The listing builds one solid part. Answer for the finished solid, in the listing's coordinates (mm). A direction names the side the tool comes from. Coordinates: 2 decimals unless noted, no trailing zeros. Write each loop counter-clockwise with the first axis right and the second up, starting at its lowest first coordinate (ties: lowest second). Pieces come first, ordered by that corner, then holes.
from build123d import *

# Parameters (mm, degrees)
SKETCH1_W             = 32
SKETCH1_H             = 32
BOSS_EXTRUDE1_DEPTH   = 4
SKETCH2_R             = 2
CUT_EXTRUDE1_DEPTH    = 3
CHAMFER1_SIZE         = 2
CHAMFER1_SIZE2        = 1.154700538
CHAMFER1_PART_2_SIZE  = 2
CHAMFER1_PART_2_SIZE2 = 1.154700538
CHAMFER1_PART_3_SIZE  = 2
CHAMFER1_PART_3_SIZE2 = 1.154700538
CHAMFER1_PART_4_SIZE  = 2
CHAMFER1_PART_4_SIZE2 = 1.154700538


with BuildPart() as part:
    # Sketch1 → Boss-Extrude1 (new body)
    with BuildSketch(Plane(origin=(0, 0, 0), x_dir=(1, 0, 0), z_dir=(0, 1, 0))):
        Rectangle(SKETCH1_W, SKETCH1_H)
    extrude(amount=BOSS_EXTRUDE1_DEPTH)

    # Sketch2 → Cut-Extrude1 (cut)
    with BuildSketch(Plane(origin=(0, 4, 0), x_dir=(1, 0, 0), z_dir=(0, 1, 0))):
        with Locations((-11.75, 11.75)):
            Circle(SKETCH2_R)
        with Locations((11.75, 11.75)):
            Circle(SKETCH2_R)
        with Locations((11.75, -11.75)):
            Circle(SKETCH2_R)
        with Locations((-11.75, -11.75)):
            Circle(SKETCH2_R)
    extrude(amount=-CUT_EXTRUDE1_DEPTH, mode=Mode.SUBTRACT)

    # Chamfer1
    chamfer1_edges = [part.edges().sort_by_distance(p)[0] for p in [
        (-16, 4, 0),
    ]]
    chamfer1_side = [part.faces().sort_by_distance(p)[0] for p in [
        (-16, 2, 0),
    ]]
    chamfer(chamfer1_edges, length=CHAMFER1_SIZE, length2=CHAMFER1_SIZE2, reference=chamfer1_side[0])

    # Chamfer1 part 2
    chamfer1_part_2_edges = [part.edges().sort_by_distance(p)[0] for p in [
        (0, 4, 16),
    ]]
    chamfer1_part_2_side = [part.faces().sort_by_distance(p)[0] for p in [
        (0, 2, 16),
    ]]
    chamfer(chamfer1_part_2_edges, length=CHAMFER1_PART_2_SIZE, length2=CHAMFER1_PART_2_SIZE2, reference=chamfer1_part_2_side[0])

    # Chamfer1 part 3
    chamfer1_part_3_edges = [part.edges().sort_by_distance(p)[0] for p in [
        (16, 4, 0),
    ]]
    chamfer1_part_3_side = [part.faces().sort_by_distance(p)[0] for p in [
        (16, 2, 0),
    ]]
    chamfer(chamfer1_part_3_edges, length=CHAMFER1_PART_3_SIZE, length2=CHAMFER1_PART_3_SIZE2, reference=chamfer1_part_3_side[0])

    # Chamfer1 part 4
    chamfer1_part_4_edges = [part.edges().sort_by_distance(p)[0] for p in [
        (0, 4, -16),
    ]]
    chamfer1_part_4_side = [part.faces().sort_by_distance(p)[0] for p in [
        (0, 2, -16),
    ]]
    chamfer(chamfer1_part_4_edges, length=CHAMFER1_PART_4_SIZE, length2=CHAMFER1_PART_4_SIZE2, reference=chamfer1_part_4_side[0])


solid = part.part
Q1. Find the intervals of material crossed by probe 1 along X at (y, z) = (1.85, -11.75); probe 2 along Z at (x, y) = (11.75, 2.4); probe 3 along X at (y, z) = (3.25, -12.5), in increasing order.
Answers below:
probe 1: x = -16 to -13.75, -9.75 to 9.75, 13.75 to 16
probe 2: z = -15.77 to -13.75, -9.75 to 9.75, 13.75 to 15.77
probe 3: x = -15.28 to -13.6, -9.9 to 9.9, 13.6 to 15.28
Q2. The part is cut by section A-A, the plane y = 3.1. Write down the section's boundary in (x, z).
Answers below:
outline: (-15.36, -15.36) - (15.36, -15.36) - (15.36, 15.36) - (-15.36, 15.36) - close; hole circle Ø4 at (-11.75, -11.75); hole circle Ø4 at (-11.75, 11.75); hole circle Ø4 at (11.75, -11.75); hole circle Ø4 at (11.75, 11.75)
Q3. The part is cut by section D-D, the plane x = 11.75. Write down the section's boundary in (y, z), then the cut area to 3 significant figures.
Answers below:
outline: (0, -16) - (2, -16) - (4, -14.85) - (4, -13.75) - (1, -13.75) - (1, -9.75) - (4, -9.75) - (4, 9.75) - (1, 9.75) - (1, 13.75) - (4, 13.75) - (4, 14.85) - (2, 16) - (0, 16) - close
area: 102 mm2
Q4. Which of the six approach directions +Z, -Z, +X, -X, +Y, -Y give full straight-line access (tool end or side, diameter ignored) to faces 1 (the face through (-12, 1, -12)), 2 (the face through (0, 1, 16))?
Answers below:
face 1: +Y
face 2: +Z, +X, -X, +Y, -Y
Q5. The part is cut by section C-C, the plane z = -11.75. Write down the section's boundary in (x, y), then the cut area to 3 significant figures.
Answers below:
outline: (-16, 0) - (16, 0) - (16, 2) - (14.85, 4) - (13.75, 4) - (13.75, 1) - (9.75, 1) - (9.75, 4) - (-9.75, 4) - (-9.75, 1) - (-13.75, 1) - (-13.75, 4) - (-14.85, 4) - (-16, 2) - close
area: 102 mm2
Q6. Given pin 1 (3 mm diameter, centred on x = 11.75, z = -11.75, fed in from +Y); pin 2 (1 mm diameter, centred on x = 7, y = 3.5, fed in from -Z), each flat-ended and moving along its own axis, determine where each tip first touches the part or whether it passes through.
Answers below:
pin 1: stops at y = 1
pin 2: stops at z = -15.42
Q7. The part is cut by section B-B, the plane x = 2.5. Write down the section's boundary in (y, z), then the cut area to 3 significant figures.
Answers below:
outline: (0, -16) - (2, -16) - (4, -14.85) - (4, 14.85) - (2, 16) - (0, 16) - close
area: 126 mm2
